Build history of the part. All positions in model axes, mm. Face numbers are marked on the shaded views. A direction names the side the tool comes from. Round coordinates to 2 decimals unless told otherwise and drop trailing zeros. Write each loop counter-clockwise with the first axis right and the second up, starting at its lowest first coordinate (ties: lowest second). Pieces come first, ordered by that corner, then holes. Notation, with made-up numbers: (5.5, 57) - (57.5, 57) arc R24 cw to (57.5, 85) - close; hole circle Ø1 at (83, 57.25). An arc over 180 degrees is marked (long way). Write each question's results on one line, items separated by ' | '.
from build123d import *

# Parameters (mm, degrees)
SKETCH_W     = 135
SKETCH_H     = 21
SKETCH_R     = 0.5
PAD_DEPTH    = 1.5
SKETCH001_W  = 97
SKETCH001_H  = 12
PAD001_DEPTH = 9
SKETCH002_W  = 10
SKETCH002_H  = 8
PAD002_DEPTH = 10
PAD003_DEPTH = 8


with BuildPart() as part:
    # Sketch → Pad (new body)
    with BuildSketch(Plane.XY):
        with Locations((0, 10.5)):
            Rectangle(SKETCH_W, SKETCH_H)
        with Locations((-64.5, 3)):
            Circle(SKETCH_R, mode=Mode.SUBTRACT)
        with Locations((64.5, 3)):
            Circle(SKETCH_R, mode=Mode.SUBTRACT)
    extrude(amount=PAD_DEPTH)

    # Sketch001 (on Face8 of Pad) → Pad001 (join)
    with BuildSketch(Plane.XY.offset(1.5)):
        with Locations((13, 12)):
            Rectangle(SKETCH001_W, SKETCH001_H)
    extrude(amount=PAD001_DEPTH)

    # Sketch002 (on Face5 of Pad001) → Pad002 (join)
    with BuildSketch(Plane.XY.offset(1.5)):
        with Locations((-54.5, 5)):
            Rectangle(SKETCH002_W, SKETCH002_H)
    extrude(amount=PAD002_DEPTH)

    # Sketch003 (on Face5 of Pad002) → Pad003 (join)
    with BuildSketch(Plane.XY.offset(1.5)):
        Polygon((-54.5, 10), (-48.5, 10), (-48.5, 2), (-38.5, 2), (-38.5, 19), (-54.5, 19), align=None)
    extrude(amount=PAD003_DEPTH)


solid = part.part
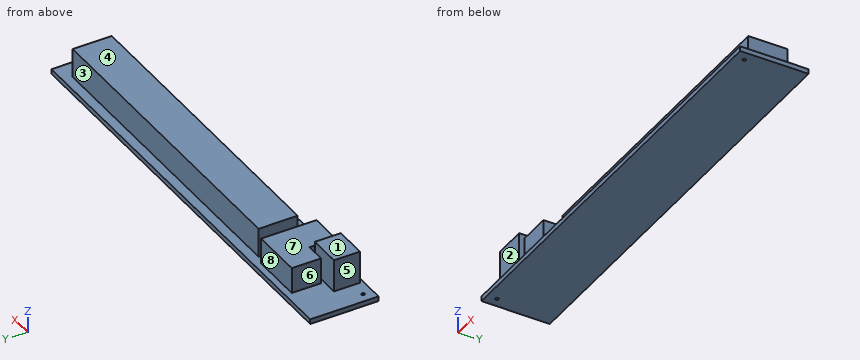
(1) Slice it at B-B, the plane z = 3.75. Write the cut outline in (x, y), and give its area (3 significant figures).
Worked answers:
outline: (-59.5, 1) - (-49.5, 1) - (-49.5, 9) - (-59.5, 9) - close; (-54.5, 10) - (-48.5, 10) - (-48.5, 2) - (-38.5, 2) - (-38.5, 19) - (-54.5, 19) - close; (-35.5, 6) - (61.5, 6) - (61.5, 18) - (-35.5, 18) - close | area: 1,470 mm2
(2) Slice it at A-A, the plane y = 13.75. Write the cut outline in (x, z), and give its area (3 significant figures).
Worked answers:
outline: (-67.5, 0) - (67.5, 0) - (67.5, 1.5) - (61.5, 1.5) - (61.5, 10.5) - (-35.5, 10.5) - (-35.5, 1.5) - (-38.5, 1.5) - (-38.5, 9.5) - (-54.5, 9.5) - (-54.5, 1.5) - (-67.5, 1.5) - close | area: 1,200 mm2
(3) Drill centre lines: probe 1 along X at (y, z) = (6.25, 7.5); probe 2 along X at (y, z) = (4, 3.25); probe 3 along Y at (x, z) = (-64.5, 1.2). Where is each one in solid material? Low to high. Write a range as [from, to].
Worked answers:
probe 1: x = [-59.5, -49.5], [-48.5, -38.5], [-35.5, 61.5] | probe 2: x = [-59.5, -49.5], [-48.5, -38.5] | probe 3: y = [0, 2.5], [3.5, 21]
(4) Two-plate mould, pull along X, no slides. Class the marked faces 6, 7 and 8: released by +X, released by -X, zero draft, split by the parting line, or undercut.
Worked answers:
face 6: released by -X | face 7: undercut | face 8: zero draft
(5) Tool access for the marked faces 1, 2, 3, 4 and 5: list every direction of +Z, -Z, +X, -X, +Y, -Y with a clear straight run to the whole face (end or side of a thin tool).
Worked answers:
face 1: +Z, +X, -X, +Y, -Y | face 2: +Z, +X, -X, -Y | face 3: +Z, +X, +Y | face 4: +Z, +X, +Y, -Y | face 5: +Z, -X, +Y, -Y
(6) Slice it at C-C, the plane x = 43. Write the cut outline in (y, z).
Worked answers:
outline: (0, 0) - (21, 0) - (21, 1.5) - (18, 1.5) - (18, 10.5) - (6, 10.5) - (6, 1.5) - (0, 1.5) - close
(7) Flat gauge pins, fed straight in: pin 1 Ø2 at (x, y) = (16.5, 11) entering from +Z; pin 2 Ø5 at (x, z) = (-4.5, 5) entering from -Y; pin 3 Ø4.5 at (x, z) = (21.5, 7) entering from +Y. Where does each tip first touch, or does it go through?
Worked answers:
pin 1: stops at z = 10.5 | pin 2: stops at y = 6 | pin 3: stops at y = 18
